The figure shows three views and two pictorial views of one solid part (mm, origin at its lowest corner). Answer the questions. Round coordinates to 2 decimals unless told otherwise and drop trailing zeros. Order: outer loops, then holes, each group sorted by start corner. A loop starts at its lowest first (then second) coordinate and runs counter-clockwise, first axis right, second up. Notation, with made-up numbers: (-13, 83) -> (10, 83) arc R17 ccw to (10, 115) -> close; hole circle Ø9 at (-27.5, 86.25). An arc over 180 degrees is marked (long way). Return JSON: item names as keys, results as strings. Group by question number.
(1) The part is cut by section A-A (x = 76.2). Determine the outline of the cut face in (y, z) (1 decimal).
(2) Consider line 1 (X direction, y = 19, z = 0.5) (1 decimal); line 2 (X direction, y = 48, z = 2.45); line 3 (X direction, y = 16.5, z = 2) (1 decimal). Determine where each line is inside the solid, lowest interval first. Write a range as [from, to].
(3) This flat-tipped pin is pushed along its axis until it touches: pin 1 (4 mm diameter, centred on x = 47.625, y = 19.05, fed in from +Z). Where does it stop, or does it pass through?
(4) The part is cut by section C-C (z = 2.4). Count the separate pieces of the cut face and the enclosed holes in it, plus the area to 3 significant figures.
(5) The part is cut by section B-B (y = 32). Determine the outline of the cut face in (x, z) (1 decimal), plus the area to 3 significant figures.
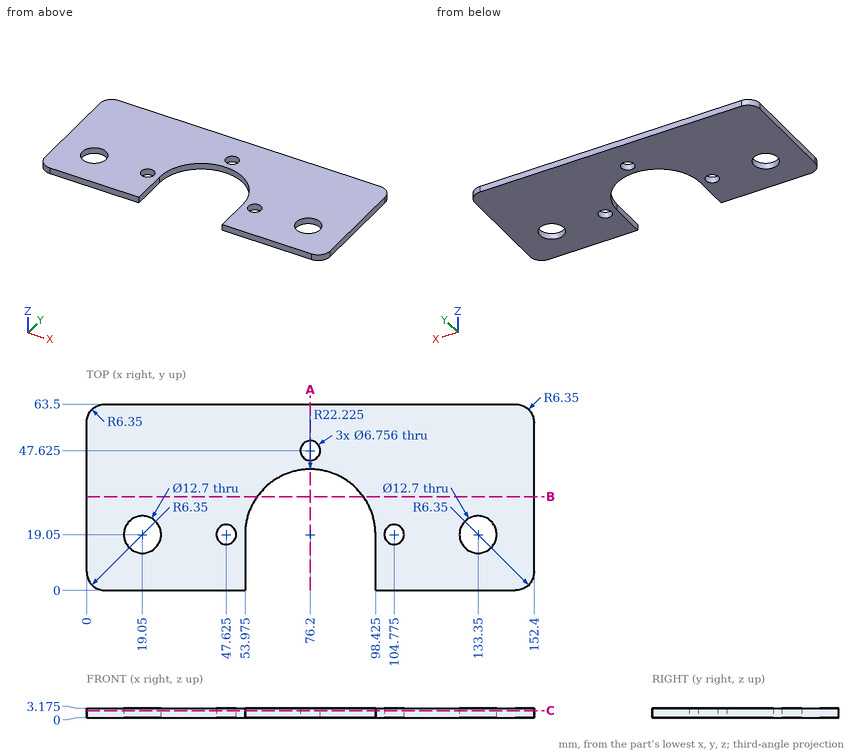
Answer below:
{
 "1": {"outline": "(41.3, 0) -> (44.2, 0) -> (44.2, 3.2) -> (41.3, 3.2) -> close; (51, 0) -> (63.5, 0) -> (63.5, 3.2) -> (51, 3.2) -> close"},
 "2": {"line 1": "x = [0, 12.7], [25.4, 44.2], [51, 54], [98.4, 101.4], [108.2, 127], [139.7, 152.4]", "line 2": "x = [0, 72.84], [79.56, 152.4]", "line 3": "x = [0, 13.2], [24.9, 45.4], [49.8, 54], [98.4, 102.6], [107, 127.5], [139.2, 152.4]"},
 "3": {"pin 1": "passes through"},
 "4": {"separate pieces": "1", "enclosed holes": "5", "area": "7,660 mm²"},
 "5": {"outline": "(0, 0) -> (58.1, 0) -> (58.1, 3.2) -> (0, 3.2) -> close; (94.3, 0) -> (152.4, 0) -> (152.4, 3.2) -> (94.3, 3.2) -> close", "area": "369 mm²"}
}
